```python
from build123d import *

# Parameters (mm, degrees)
SKETCH1_R           = 4
SKETCH1_W           = 5.6
SKETCH1_H           = 20.6
BOSS_EXTRUDE1_DEPTH = 5


with BuildPart() as part:
    # Sketch1 → Boss-Extrude1 (new body)
    with BuildSketch(Plane.XY):
        Polygon((0, 0), (100, 0), (100, 60), (60.3, 60), (60.3, 54.7), (39.7, 54.7), (39.7, 60), (0, 60), align=None)
        with Locations((25, 45)):
            Circle(SKETCH1_R, mode=Mode.SUBTRACT)
        with Locations((42, 45)):
            Circle(SKETCH1_R, mode=Mode.SUBTRACT)
        with Locations((59, 45)):
            Circle(SKETCH1_R, mode=Mode.SUBTRACT)
        with Locations((76, 45)):
            Circle(SKETCH1_R, mode=Mode.SUBTRACT)
        with Locations((42, 30)):
            Circle(SKETCH1_R, mode=Mode.SUBTRACT)
        with Locations((59, 30)):
            Circle(SKETCH1_R, mode=Mode.SUBTRACT)
        with Locations((76, 30)):
            Circle(SKETCH1_R, mode=Mode.SUBTRACT)
        with Locations((42, 15)):
            Circle(SKETCH1_R, mode=Mode.SUBTRACT)
        with Locations((59, 15)):
            Circle(SKETCH1_R, mode=Mode.SUBTRACT)
        with Locations((76, 15)):
            Circle(SKETCH1_R, mode=Mode.SUBTRACT)
        with Locations((25, 30)):
            Circle(SKETCH1_R, mode=Mode.SUBTRACT)
        with Locations((25, 15)):
            Circle(SKETCH1_R, mode=Mode.SUBTRACT)
        with Locations((12.5, 20)):
            Rectangle(SKETCH1_W, SKETCH1_H, mode=Mode.SUBTRACT)
        with Locations((87.5, 20)):
            Rectangle(SKETCH1_W, SKETCH1_H, mode=Mode.SUBTRACT)
    extrude(amount=BOSS_EXTRUDE1_DEPTH)


solid = part.part
```
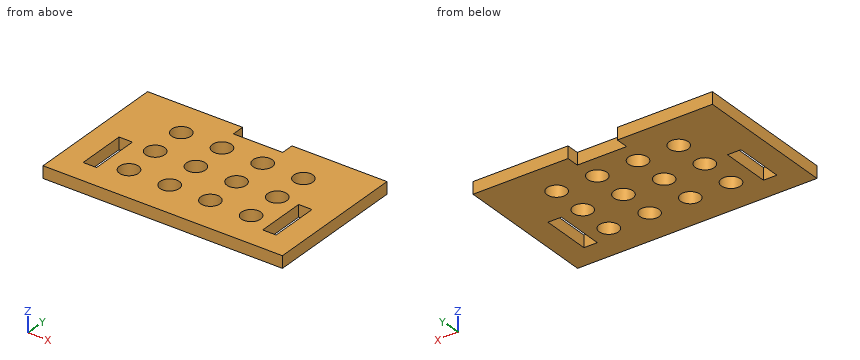
Source: CAD feature listing. Evaluate the final solid. Frame: model axes, mm. Coordinates: 2 decimals unless noted, no trailing zeros. Write each loop counter-clockwise with the first axis right and the second up, starting at its lowest first coordinate (ties: lowest second). Pieces come first, ordered by that corner, then holes. Notation, with made-up numbers: (41.5, 68.5) - (89.5, 68.5) arc R31 cw to (89.5, 107.5) - close; hole circle Ø2 at (71.25, -3). An arc over 180 degrees is marked (long way). Answer as a JSON object with one key per item and string values.
Q1. Section query D-D, the plane y = 56. Output: boundary loops of the cut face in (x, z), plus the area to 3 significant figures.
Ans:
{"outline": "(0, 0) - (39.7, 0) - (39.7, 5) - (0, 5) - close; (60.3, 0) - (100, 0) - (100, 5) - (60.3, 5) - close", "area": "397 mm2"}
Q2. Section query A-A, the plane x = 59. Output: boundary loops of the cut face in (y, z).
Ans:
{"outline": "(0, 0) - (11, 0) - (11, 5) - (0, 5) - close; (19, 0) - (26, 0) - (26, 5) - (19, 5) - close; (34, 0) - (41, 0) - (41, 5) - (34, 5) - close; (49, 0) - (54.7, 0) - (54.7, 5) - (49, 5) - close"}
Q3. Material intervals for line 1 (Y direction, x = 42, z = 2.8); line 2 (Y direction, x = 25, z = 4); line 3 (Y direction, x = 12.5, z = 1.45), sorted ascending. Write a range as [from, to].
Ans:
{"line 1": "y = [0, 11], [19, 26], [34, 41], [49, 54.7]", "line 2": "y = [0, 11], [19, 26], [34, 41], [49, 60]", "line 3": "y = [0, 9.7], [30.3, 60]"}
Q4. Section query C-C, the plane z = 3.2. State how many separate pieces and enclosed holes the cut face has, plus the area to 3 significant figures.
Ans:
{"separate pieces": "1", "enclosed holes": "14", "area": "5,060 mm2"}
Q5. Section query B-B, the plane y = 45. Output: boundary loops of the cut face in (x, z), plus the area to 3 significant figures.
Ans:
{"outline": "(0, 0) - (21, 0) - (21, 5) - (0, 5) - close; (29, 0) - (38, 0) - (38, 5) - (29, 5) - close; (46, 0) - (55, 0) - (55, 5) - (46, 5) - close; (63, 0) - (72, 0) - (72, 5) - (63, 5) - close; (80, 0) - (100, 0) - (100, 5) - (80, 5) - close", "area": "340 mm2"}
